Design review of the part built by this model. Coordinates are the model's own, in mm. Face numbers are marked on the shaded views. A direction names the side the tool comes from. Coordinates: 2 decimals unless noted, no trailing zeros. Write each loop counter-clockwise with the first axis right and the second up, starting at its lowest first coordinate (ties: lowest second). Pieces come first, ordered by that corner, then holes. Notation, with made-up numbers: (26, 68.25) - (59, 68.25) arc R10 ccw to (59, 80.25) - close; hole circle Ø9 at (88, 35). An arc over 180 degrees is marked (long way). One line per item, written item: value.
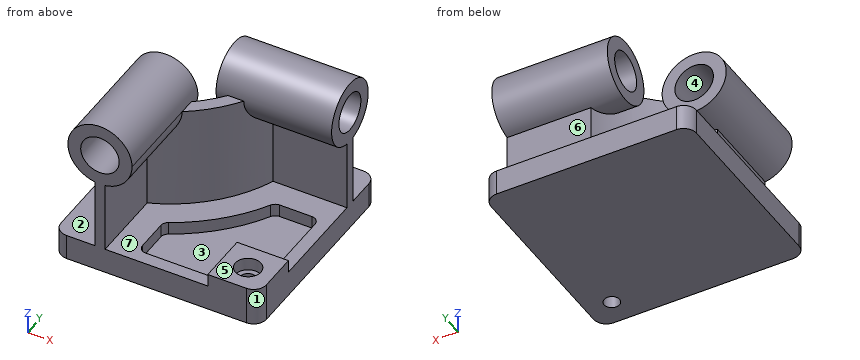
Autodesk Fusion 360 part; units mm, degrees
sketch "Sketch1" plane through (0, 0, 0) normal (0, 0, 1) x (1, 0, 0)
  line L0 (20, -20) -> (-20, -20)
  line L1 (-20, -20) -> (-20, 20)
  line L2 (-20, 20) -> (20, 20)
  line L3 (20, 20) -> (20, -20)
  line L4 (-20, -20) -> (20, 20) construction
  line L5 (20, -20) -> (10, -20)
  line L6 (10, -20) -> (10, -10)
  line L7 (10, -10) -> (20, -10)
  line L8 (20, -10) -> (20, -20)
  line L9 (-12, -20) -> (-12, -3.6854)
  line L10 (3.6854, 12) -> (20, 12)
  line L11 (-10, -20) -> (-10, -5.6174)
  line L12 (5.6174, 10) -> (20, 10)
  arc A0 (-10, -5.6174) -> (5.6174, 10) centre (-20, 20) ccw
  arc A1 (-12, -3.6854) -> (3.6854, 12) centre (-20, 20) ccw
  line L13 (20, -20) -> (-2.3223, 2.3223) construction
  line L14 (-10, 10) -> (-20, 20) construction
  line L15 (17.5, 5) -> (17.5, -10)
  line L16 (10, -17.5) -> (-5, -17.5)
  line L17 (-5, -17.5) -> (-5, -8.8314)
  arc A2 (-5, -8.8314) -> (8.8314, 5) centre (-20, 20) ccw
  line L18 (8.8314, 5) -> (17.5, 5)
  circle A3 centre (15, -15) radius 2.5
  circle A4 centre (15, -15) radius 1.5
  dimension "d1" = 40
  dimension "d2" = 40
  dimension "d3" = 10
  dimension "d4" = 10
  dimension "d5" = 50
  dimension "d6" = 55
  dimension "d7" = 8
  dimension "d9" = 2.5
  dimension "d10" = 2.5
  dimension "d12" = 5
  dimension "d13" = 3
  dimension "d14" = 5
extrude "Extrude1" add sketch "Sketch1" against normal blind 5 contours L0 L3 L5 L6 L7 L8 | L0 L3 L6 L7 L11 L12 A0 L15 L16 L17 A2 L18 | L0 L3 L9 L10 L11 L12 A0 A1 | L6 L7 L15 L16 L17 A2 L18 | L0 L1 L2 L3 L9 L10 A1 | A3 | A4
extrude "Extrude2" cut sketch "Sketch1" against normal blind 2.5 contours L6 L7 L15 L16 L17 A2 L18
extrude "Extrude3" cut sketch "Sketch1" against normal blind 17 contours A4
extrude "Extrude4" add sketch "Sketch1" along normal blind 2.5 contours L0 L3 L5 L6 L7 L8
extrude "Extrude5" add sketch "Sketch1" along normal blind 20 contours L0 L3 L9 L10 L11 L12 A0 A1
fillet "Fillet1" radius 2.5 4 edges at (20, -20, -1.25) (20, 20, -2.5) (-20, -20, -2.5) (-20, 20, -2.5)
fillet "Fillet2" radius 1.5 4 edges at (-5, -8.8314, -1.25) (8.8314, 5, -1.25) (-5, -17.5, -1.25) (17.5, 5, -1.25)
sketch "Sketch2" plane through (0, -20, 0) normal (0, -1, 0) x (1, 0, 0)
  line L0 (-17.5, 0) -> (-17.5, -5)
  line L1 (-17.5, -5) -> (17.5, -5)
  line L2 (17.5, -5) -> (17.5, 2.5)
  line L3 (17.5, 2.5) -> (10, 2.5)
  line L4 (10, 2.5) -> (10, 0)
  line L5 (10, 0) -> (-10, 0)
  line L6 (-10, 0) -> (-10, 20)
  line L7 (-10, 20) -> (-12, 20)
  line L8 (-12, 20) -> (-12, 0)
  line L9 (-12, 0) -> (-17.5, 0)
  circle A0 centre (-11, 20) radius 6.25
  dimension "d29" = 12.5
extrude "Extrude6" add sketch "Sketch2" against normal blind 22.5 contours L6 L7 L8 A0 | L6 L7 L8 A0
sketch "Sketch3" plane through (20, 0, 0) normal (1, 0, 0) x (0, 1, 0)
  line L0 (17.5, -5) -> (17.5, 0)
  line L1 (17.5, 0) -> (12, 0)
  line L2 (12, 0) -> (12, 20)
  line L3 (12, 20) -> (10, 20)
  line L4 (10, 20) -> (10, 0)
  line L5 (10, 0) -> (-10, 0)
  line L6 (-10, 0) -> (-10, 2.5)
  line L7 (-10, 2.5) -> (-17.5, 2.5)
  line L8 (-17.5, 2.5) -> (-17.5, -5)
  line L9 (-17.5, -5) -> (17.5, -5)
  circle A0 centre (11, 20) radius 6.25
  dimension "d32" = 12.5
extrude "Extrude7" add sketch "Sketch3" against normal blind 22.5 contours L2 L3 L4 A0 | L2 L3 L4 A0
hole "Hole1" at (-11, -20, 20) direction (0, 1, 0) diameter 7.5 end through all
hole "Hole2" at (20, 11, 20) direction (-1, 0, 0) diameter 7.5 end through all
1. Consider section C-C, the plane x = 15. Write out the cut boundary in (y, z).
Answer block:
outline: (-20, -5) - (-16.5, -5) - (-16.5, 0) - (-17.5, 0) - (-17.5, 2.5) - (-20, 2.5) - close; (-13.5, -5) - (20, -5) - (20, 0) - (12, 0) - (12, 13.83) arc R6.25 ccw (long way) to (10, 13.83) - (10, 0) - (5, 0) - (5, -2.5) - (-10, -2.5) - (-10, 2.5) - (-12.5, 2.5) - (-12.5, 0) - (-13.5, 0) - close; hole circle Ø7.5 at (11, 20)
2. Mouldability with a two-part tool opening along X and no side actions: class the marked faces 1, 2, 3 and 4 as released by +X, released by -X, zero draft, split by the parting line, or undercut.
Answer block:
face 1: released by +X
face 2: zero draft
face 3: undercut
face 4: undercut
3. For the marked faces 5, 6 and 7, list the 3-axis set-ups (+Z, -Z, +X, -X, +Y, -Y) from which the entire face can be reached by the end or side of a thin tool; tool diameter is ignored.
Answer block:
face 5: +Z, +X, -Y
face 6: +X, -X, +Y
face 7: none
4. Consider section B-B, the plane z = 1.5. Write out the cut boundary in (x, y).
Answer block:
outline: (-12, -20) - (-10, -20) - (-10, -5.62) arc R27.5 ccw to (5.62, 10) - (20, 10) - (20, 12) - (3.69, 12) arc R25 cw to (-12, -3.69) - close; (10, -20) - (17.5, -20) arc R2.5 ccw to (20, -17.5) - (20, -10) - (10, -10) - close; hole circle Ø5 at (15, -15)
5. Wall thickness on line 1 along Y through (x, z) = (15, -1.6); line 2 along Y through (x, z) = (15, 1); line 3 along Z through (x, y) = (-2, 6): over which ranges is each line inside the solid? List them lowest first.
Answer block:
line 1: y = -20 to -16.5, -13.5 to -10, 5 to 20
line 2: y = -20 to -17.5, -12.5 to -10, 10 to 12
line 3: z = -5 to 0, 16.25 to 23.75
6. Insertion check: pin 1 Ø12 at (y, z) = (-6, 18.5) entering from -X; pin 2 Ø6 at (y, z) = (9.5, 20.5) entering from -X; pin 3 Ø7 at (y, z) = (-14.5, 4.5) entering from +X; pin 4 Ø1.5 at (x, y) = (-8.5, -15.5) entering from +Z. Each pin has a flat end and moves straight along its axis. Give the tip position at first contact, or say it passes through.
Answer block:
pin 1: stops at x = -17.25
pin 2: stops at x = -2.5
pin 3: stops at x = 20
pin 4: stops at z = 26
7. Consider section D-D, the plane z = 18.5. Write out the cut boundary in (x, y), then the cut area to 3 significant figures.
Answer block:
outline: (-17.07, -20) - (-14.44, -20) - (-14.44, 2.5) - (-17.07, 2.5) - close; (-7.56, -20) - (-4.93, -20) - (-4.93, -3) arc R27.5 ccw to (3, 4.93) - (20, 4.93) - (20, 7.56) - (-2.5, 7.56) - (-2.5, 4.93) - (-0.05, 4.93) arc R25 cw to (-4.93, 0.05) - (-4.93, 2.5) - (-7.56, 2.5) - close; (-2.5, 14.44) - (20, 14.44) - (20, 17.07) - (-2.5, 17.07) - close
area: 260 mm^2
8. Consider section A-A, the plane y = -15. Write out the cut boundary in (x, z).
Answer block:
outline: (-20, -5) - (13.5, -5) - (13.5, 0) - (12.5, 0) - (12.5, 2.5) - (10, 2.5) - (10, -2.5) - (-5, -2.5) - (-5, 0) - (-10, 0) - (-10, 13.83) arc R6.25 ccw (long way) to (-12, 13.83) - (-12, 0) - (-20, 0) - close; (16.5, -5) - (20, -5) - (20, 2.5) - (17.5, 2.5) - (17.5, 0) - (16.5, 0) - close; hole circle Ø7.5 at (-11, 20)
